Part model, mm, in its own coordinate system. A direction names the side the tool comes from. Give positions to 0.01 mm unless a question says otherwise; leave off trailing zeros. Write each loop counter-clockwise with the first axis right and the second up, starting at its lowest first coordinate (ties: lowest second). Pieces come first, ordered by that corner, then holes. Notation, with made-up numbers: M 76,-11.5 L 122,-11.5 A19 cw 122,12.5 Z; hole C -39.75,5 d2. An arc over 180 degrees is marked long. Use a Markdown table: item, result.
```python
from build123d import *

# Parameters (mm, degrees)
F1_DEPTH = 50.8
F2_W     = 55.727891
F2_H     = 82.951285
F3_DEPTH = 25.4
F4_R     = 6.803982
F4_R_2   = 7.03444
F4_R_3   = 7.085439
F4_R_4   = 7.921759
F5_DEPTH = 63.5
F6_W     = 29.292612
F6_H     = 16.20914
F7_DEPTH = 174.244


with BuildPart() as f1:
    # F0 (on Front) → F1 (new body, symmetric)
    with BuildSketch(Plane.XZ):
        Polygon((11.369772, 55.651672), (-97.532384, 55.651672), (-97.532384, -55.651672), (18.7361, -55.651672), (18.7361, -35.870828), (97.532384, -35.870828), align=None)
    extrude(amount=F1_DEPTH, both=True)

    # F2 (on face) → F3 (cut)
    with BuildSketch(Plane.XZ.offset(50.8)):
        with Locations((70.620689, 5.604814)):
            Rectangle(F2_W, F2_H)
    extrude(amount=-F3_DEPTH, mode=Mode.SUBTRACT)

    # F4 (on Top) → F5 (cut, symmetric)
    with BuildSketch(Plane.XY):
        with Locations((34.800593, 31.432793)):
            Circle(F4_R)
        with Locations((35.442077, -3.207429)):
            Circle(F4_R_2)
        with Locations((73.28973, 33.998735)):
            Circle(F4_R_3)
        with Locations((75.855672, -2.886686)):
            Circle(F4_R_4)
    extrude(amount=F5_DEPTH, both=True, mode=Mode.SUBTRACT)

    # F6 (on face) → F7 (cut)
    with BuildSketch(Plane(origin=(-97.532384, 0, 0), x_dir=(0, -1, 0), z_dir=(-1, 0, 0))):
        with Locations((0, 47.547102)):
            Rectangle(F6_W, F6_H)
    extrude(amount=-F7_DEPTH, mode=Mode.SUBTRACT)


solid = f1.part
```
1. Cut at B-B, the plane z = 43.5. Give the cut face in (x, y), then the cut area to 3 significant figures.
Findings below:
| item | result |
|---|---|
| outline | M -97.53,-50.8 L 22.81,-50.8 L 22.81,-14.65 L -97.53,-14.65 Z; M -97.53,14.65 L 22.81,14.65 L 22.81,50.8 L -97.53,50.8 Z |
| area | 8,700 mm2 |
2. Two-plate mould, pull along Y, no slides. Class faces 5 (the cylindrical face through (67.94, -2.54, -23.29)), 6 (the flat face through (58, -25.4, -19)), 7 (the flat face through (-97.532, -1, 1)): released by +Y, released by -Y, zero draft, split by the parting line, or undercut.
Findings below:
| item | result |
|---|---|
| face 5 | undercut |
| face 6 | released by -Y |
| face 7 | zero draft |
3. Cut at C-C, the plane x = -65. Give the cut face in (y, z).
Findings below:
| item | result |
|---|---|
| outline | M -50.8,-55.65 L 50.8,-55.65 L 50.8,55.65 L 14.65,55.65 L 14.65,39.44 L -14.65,39.44 L -14.65,55.65 L -50.8,55.65 Z |
4. Cut at D-D, the plane x = 76.5. Give the cut face in (y, z), then the cut area to 3 significant figures.
Findings below:
| item | result |
|---|---|
| outline | M -25.4,-35.87 L -10.78,-35.87 L -10.78,-13.53 L -25.4,-13.53 Z; M 5.01,-35.87 L 27.68,-35.87 L 27.68,-13.53 L 5.01,-13.53 Z; M 40.32,-35.87 L 50.8,-35.87 L 50.8,-13.53 L 40.32,-13.53 Z |
| area | 1,070 mm2 |
5. Drill centre lines: L1, parallel to Y at x = 35, z = -22; L2, parallel to Y at x = -80, z = 40; L3, parallel to X at y = 30.5, z = -25. Where is each one in solid material? Low to high.
Findings below:
| item | result |
|---|---|
| L1 | -50.8 to -10.23, 3.81 to 24.63, 38.23 to 50.8 |
| L2 | -50.8 to -14.65, 14.65 to 50.8 |
| L3 | -97.53 to 28.06, 41.54 to 67.13, 79.45 to 87.3 |
6. Cut at A-A, the plane y = -32. Give the cut face in (x, z).
Findings below:
| item | result |
|---|---|
| outline | M -97.53,-55.65 L 18.74,-55.65 L 18.74,-35.87 L 42.76,-35.87 L 42.76,22.31 L 11.37,55.65 L -97.53,55.65 Z |
7. Tool access for faces 1 (the flat face through (-36, -14.646, 47)), 2 (the flat face through (42.757, -38, -7)), 3 (the flat face through (58, -1, -35.871)), 4 (the flat face through (-23, 50.8, 1)): list every direction of +Z, -Z, +X, -X, +Y, -Y with a clear straight run to the whole face (end or side of a thin tool).
Findings below:
| item | result |
|---|---|
| face 1 | +Z, +X, -X |
| face 2 | +Z, -Z, +X, -Y |
| face 3 | -Z, +X, +Y, -Y |
| face 4 | +Z, -Z, +X, -X, +Y |
8. Drop flat-ended pins along their axis: P1, Ø22.5, axis at x = 73.29, y = 34, coming from the -Z side; P2, Ø16, axis at x = 35.44, y = -3.21, coming from the +Z side; P3, Ø22, axis at y = 2, z = -49, coming from the +X side. Give the stop position or say it passes through.
Findings below:
| item | result |
|---|---|
| P1 | z = -35.87 |
| P2 | z = 38.58 |
| P3 | x = 18.74 |
